Study the drawing (mm; zero at the part's minimum x, y, z) and answer. Coordinates: 2 decimals unless noted, no trailing zeros. Loops run counter-clockwise (first coordinate to the right, second up) from the corner with the lowest first, then second, coordinate; pieces in that order, holes last.
Q1. Straight lines are drawn through the part: line 1 (Y direction, x = 71, z = 1.1) (3 decimals); line 2 (X direction, y = 123.5, z = 0.95) (3 decimals). For each, find the intervals that lie inside material, in ascending order.
Q2. Section A-A (z = 1.9) is taken. Give the vertices of the cut face in (x, y) (3 decimals), then the cut area to 3 significant figures.
Q3. Section B-B (y = 217) is taken. Give the vertices of the cut face in (x, z) (3 decimals).
Q4. Flat-ended cylindrical pins translate along their axes: P1, Ø1, axis at y = 212.5, z = 1.5, coming from the -X side (3 decimals); P2, Ø1, axis at x = 76.5, z = 1, coming from the +Y side (3 decimals); P3, Ø1, axis at x = 1.5, z = 2.5, coming from the +Y side. Find the tip coordinate at first contact, or state that the pin passes through.
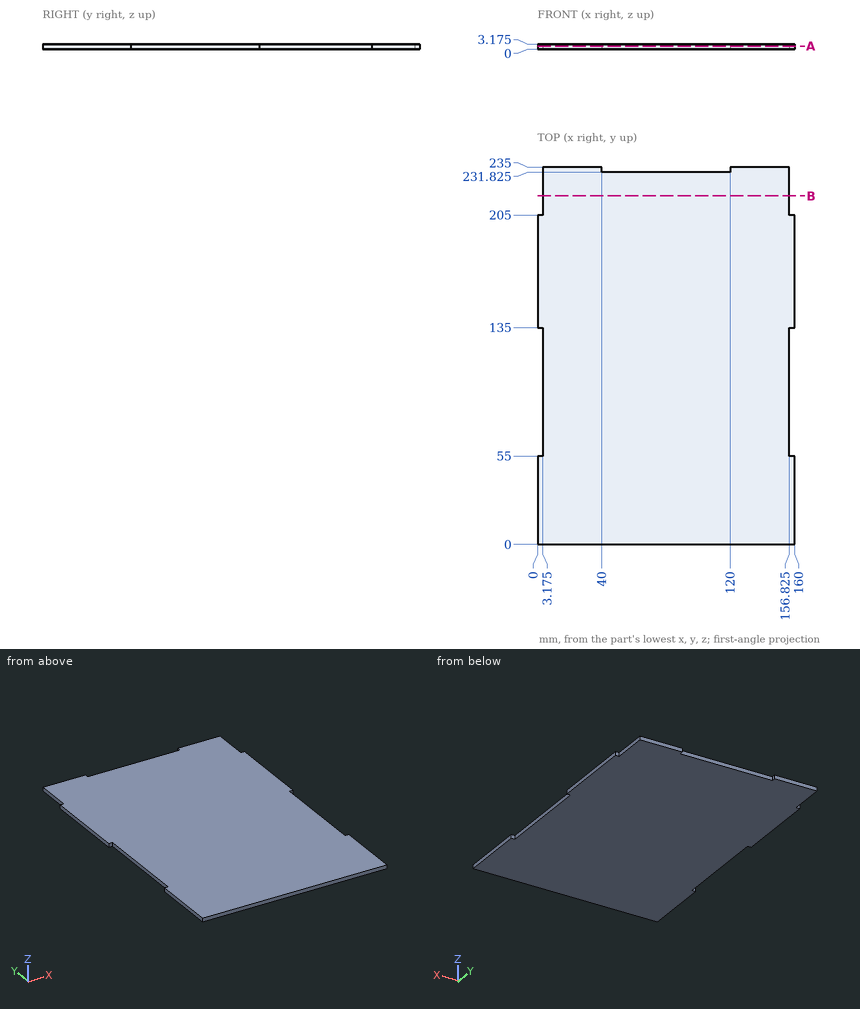
Numbers:
1. line 1: y = 0 to 231.825
1. line 2: x = 3.175 to 156.825
2. outline: (0, 0) - (160, 0) - (160, 55) - (156.825, 55) - (156.825, 135) - (160, 135) - (160, 205) - (156.825, 205) - (156.825, 235) - (120, 235) - (120, 231.825) - (40, 231.825) - (40, 235) - (3.175, 235) - (3.175, 205) - (0, 205) - (0, 135) - (3.175, 135) - (3.175, 55) - (0, 55) - close
2. area: 36,600 mm2
3. outline: (3.175, 0) - (156.825, 0) - (156.825, 3.175) - (3.175, 3.175) - close
4. P1: stops at x = 3.175
4. P2: stops at y = 231.825
4. P3: stops at y = 205
